```python
from build123d import *

# Parameters (mm, degrees)
SKETCH1_W           = 132
SKETCH1_H           = 160
BOSS_EXTRUDE1_DEPTH = 6
SKETCH3_W           = 32
SKETCH3_H           = 54
SKETCH3_W_2         = 26
SKETCH3_H_2         = 48
BOSS_EXTRUDE2_DEPTH = 17.5
SKETCH4_W           = 32
SKETCH4_H           = 54
BOSS_EXTRUDE3_DEPTH = 3
SKETCH5_W           = 25
SKETCH5_H           = 17
CUT_EXTRUDE1_DEPTH  = 3
SKETCH6_W           = 12
SKETCH6_H           = 54
BOSS_EXTRUDE4_DEPTH = 3
SKETCH7_R           = 1.6
CUT_EXTRUDE2_DEPTH  = 106.177231376
SKETCH8_W           = 3
SKETCH8_H           = 6.5
BOSS_EXTRUDE5_DEPTH = 20
SKETCH9_R           = 1.55
CUT_EXTRUDE3_DEPTH  = 6
SKETCH10_R          = 1.6
CUT_EXTRUDE4_DEPTH  = 108.043215572
SKETCH11_W          = 2.5
SKETCH11_H          = 7
BOSS_EXTRUDE6_DEPTH = 19.36
SKETCH12_R          = 1.6
CUT_EXTRUDE5_DEPTH  = 19.36
SKETCH13_W          = 3
SKETCH13_H          = 7
BOSS_EXTRUDE7_DEPTH = 15
SKETCH14_R          = 2
CUT_EXTRUDE6_DEPTH  = 15
CUT_EXTRUDE7_START  = -6
CUT_EXTRUDE7_DEPTH  = 6
SKETCH16_R          = 1.6
CUT_EXTRUDE8_DEPTH  = 15
CUT_EXTRUDE9_DEPTH  = 69
SKETCH18_W          = 9
SKETCH18_H          = 3
CUT_EXTRUDE10_DEPTH = 69
SKETCH19_R          = 1.55
CUT_EXTRUDE11_DEPTH = 69


# Read off the part's stored shape, not the designer's step: Cut-Extrude7
with BuildPart() as part:
    # Sketch1 → Boss-Extrude1 (new body)
    with BuildSketch(Plane.XY):
        Rectangle(SKETCH1_W, SKETCH1_H)
    extrude(amount=BOSS_EXTRUDE1_DEPTH)

    # Sketch3 → Boss-Extrude2 (add)
    with BuildSketch(Plane.XY.offset(6)):
        with Locations((0, -53)):
            Rectangle(SKETCH3_W, SKETCH3_H)
        with Locations((0, -53)):
            Rectangle(SKETCH3_W_2, SKETCH3_H_2, mode=Mode.SUBTRACT)
    extrude(amount=BOSS_EXTRUDE2_DEPTH)

    # Sketch4 → Boss-Extrude3 (add)
    with BuildSketch(Plane.XY.offset(23.5)):
        with Locations((0, -53)):
            Rectangle(SKETCH4_W, SKETCH4_H)
    extrude(amount=BOSS_EXTRUDE3_DEPTH)

    # Sketch5 → Cut-Extrude1 (cut)
    with BuildSketch(Plane.XZ.offset(80)):
        with Locations((0, 14.5)):
            Rectangle(SKETCH5_W, SKETCH5_H)
    extrude(amount=-CUT_EXTRUDE1_DEPTH, mode=Mode.SUBTRACT)

    # Sketch6 → Boss-Extrude4 (add)
    with BuildSketch(Plane.XY.offset(6)):
        with Locations((-22, -53)):
            Rectangle(SKETCH6_W, SKETCH6_H)
        with Locations((22, -53)):
            Rectangle(SKETCH6_W, SKETCH6_H)
    extrude(amount=BOSS_EXTRUDE4_DEPTH)

    # Sketch7 → Cut-Extrude2 (cut, through all)
    with BuildSketch(Plane.XY.offset(9)):
        with Locations((-22, -69)):
            Circle(SKETCH7_R)
        with Locations((-22, -33)):
            Circle(SKETCH7_R)
        with Locations(Location((22, -69, 0), (0, 0, 180))):
            Circle(SKETCH7_R)
        with Locations(Location((22, -33, 0), (0, 0, 180))):
            Circle(SKETCH7_R)
    extrude(amount=-CUT_EXTRUDE2_DEPTH, mode=Mode.SUBTRACT)

    # Sketch8 → Boss-Extrude5 (add)
    with BuildSketch(Plane.XY.offset(6)):
        with Locations((-54.38, -76.75)):
            Rectangle(SKETCH8_W, SKETCH8_H)
        with Locations((-54.38, -30.25)):
            Rectangle(SKETCH8_W, SKETCH8_H)
    boss_extrude5 = extrude(amount=BOSS_EXTRUDE5_DEPTH)

    # Sketch9 → Cut-Extrude3 (cut)
    with BuildSketch(Plane.ZY.offset(55.88)):
        with Locations((10.35, -76.75)):
            Circle(SKETCH9_R)
        with Locations((19.65, -76.75)):
            Circle(SKETCH9_R)
        with Locations((10.35, -30.25)):
            Circle(SKETCH9_R)
        with Locations((19.65, -30.25)):
            Circle(SKETCH9_R)
    cut_extrude3 = extrude(amount=-CUT_EXTRUDE3_DEPTH, mode=Mode.SUBTRACT)

    # Mirror1: Boss-Extrude5, Cut-Extrude3 across plane
    add(boss_extrude5.mirror(Plane(origin=(0, 0, 0), x_dir=(0, 0, 1), z_dir=(1, 0, 0))))
    add(cut_extrude3.mirror(Plane(origin=(0, 0, 0), x_dir=(0, 0, 1), z_dir=(1, 0, 0))), mode=Mode.SUBTRACT)

    # Sketch10 → Cut-Extrude4 (cut, through all)
    with BuildSketch(Plane(origin=(0, 0, 0), x_dir=(-1, 0, 0), z_dir=(0, 0, -1))):
        with Locations((-24.1, -75.572749788)):
            Circle(SKETCH10_R)
        with Locations((-21.15, -12.732749788)):
            Circle(SKETCH10_R)
        with Locations(Location((21.15, -12.732749788, 0), (0, 0, 180))):
            Circle(SKETCH10_R)
        with Locations((24.1, -75.572749788)):
            Circle(SKETCH10_R)
    extrude(amount=-CUT_EXTRUDE4_DEPTH, mode=Mode.SUBTRACT)

    # Sketch11 → Boss-Extrude6 (add)
    with BuildSketch(Plane(origin=(0, 0, 0), x_dir=(-1, 0, 0), z_dir=(0, 0, -1))):
        with Locations((-17.9, 1.267250212)):
            Rectangle(SKETCH11_W, SKETCH11_H)
        with Locations((-17.9, 50.267250212)):
            Rectangle(SKETCH11_W, SKETCH11_H)
    extrude(amount=BOSS_EXTRUDE6_DEPTH)

    # Sketch12 → Cut-Extrude5 (cut)
    with BuildSketch(Plane(origin=(19.15, 0, 0), x_dir=(0, 0, -1), z_dir=(1, 0, 0))):
        with Locations(Location((4.5, 50.267250212, 0), (0, 0, 90))):
            Circle(SKETCH12_R)
        with Locations(Location((14.5, 50.267250212, 0), (0, 0, 90))):
            Circle(SKETCH12_R)
        with Locations(Location((4.5, 1.267250212, 0), (0, 0, 90))):
            Circle(SKETCH12_R)
        with Locations(Location((14.5, 1.267250212, 0), (0, 0, 90))):
            Circle(SKETCH12_R)
    extrude(amount=-CUT_EXTRUDE5_DEPTH, mode=Mode.SUBTRACT)

    # Sketch13 → Boss-Extrude7 (add)
    with BuildSketch(Plane(origin=(0, 0, 0), x_dir=(-1, 0, 0), z_dir=(0, 0, -1))):
        with Locations((29.35, 35.967250212)):
            Rectangle(SKETCH13_W, SKETCH13_H)
    extrude(amount=BOSS_EXTRUDE7_DEPTH)

    # Sketch14 → Cut-Extrude6 (cut)
    with BuildSketch(Plane.ZY.offset(30.85)):
        with Locations((-9.9, 35.967250212)):
            Circle(SKETCH14_R)
    extrude(amount=-CUT_EXTRUDE6_DEPTH, mode=Mode.SUBTRACT)

    # Cut-Extrude7 outline → Cut-Extrude7 (cut)
    with BuildSketch(Plane(origin=(0, 0, 0), x_dir=(-1, 0, 0), z_dir=(0, 0, -1)).offset(CUT_EXTRUDE7_START)):
        Polygon((-30.85, 56.767250212), (30.85, 56.767250212), (30.85, -24), (58.88, -24), (58.88, -80), (66, -80), (66, 80), (-66, 80), (-66, -80), (-58.88, -80), (-58.88, -24), (-30.85, -24), align=None)
    extrude(amount=CUT_EXTRUDE7_DEPTH, mode=Mode.SUBTRACT)

    # Sketch16 → Cut-Extrude8 (cut)
    with BuildSketch(Plane(origin=(0, 0, 0), x_dir=(-1, 0, 0), z_dir=(0, 0, -1))):
        Circle(SKETCH16_R)
        with Locations((0, 52.767250212)):
            Circle(SKETCH16_R)
    extrude(amount=-CUT_EXTRUDE8_DEPTH, mode=Mode.SUBTRACT)

    # Sketch17 → Cut-Extrude9 (cut)
    with BuildSketch(Plane(origin=(0, 0, 0), x_dir=(-1, 0, 0), z_dir=(0, 0, -1))):
        Polygon((-30.85, 56.767250212), (30.85, 56.767250212), (30.85, 39.467250212), (18.85, 39.467250212), (18.85, 32.467250212), (30.85, 32.467250212), (58.88, -24), (58.88, -80), (-58.88, -80), (-58.88, 56.767250212), align=None)
    extrude(amount=-CUT_EXTRUDE9_DEPTH, mode=Mode.SUBTRACT)


with BuildPart() as body_2:
    # of the pieces the cut leaves, the one that is kept (cut_extrude9_keep)
    add(part.part.solids().sort_by_distance((-27.85, 39.467250212, 0))[0])

    # Sketch18 → Cut-Extrude10 (cut)
    with BuildSketch(Plane.XZ.offset(-32.467250212)):
        with Locations((-23.35, 1.5)):
            Rectangle(SKETCH18_W, SKETCH18_H)
    extrude(amount=-CUT_EXTRUDE10_DEPTH, mode=Mode.SUBTRACT)

    # Sketch19 → Cut-Extrude11 (cut)
    with BuildSketch(Plane(origin=(0, 0, 3), x_dir=(-1, 0, 0), z_dir=(0, 0, -1))):
        with Locations((22.35, 35.967250212)):
            Circle(SKETCH19_R)
    extrude(amount=-CUT_EXTRUDE11_DEPTH, mode=Mode.SUBTRACT)


solid = body_2.part
```
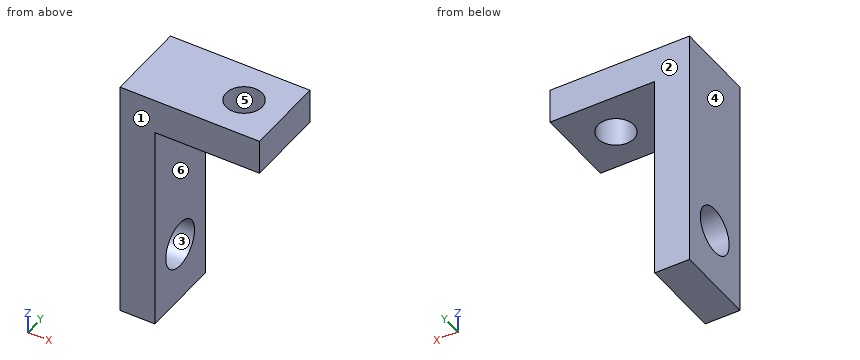
Input: part model. Units: mm. Frame: model coordinates. Face numbers are marked on the shaded views. A direction names the side the tool comes from. Coordinates: 2 decimals unless noted, no trailing zeros. Write each loop counter-clockwise with the first axis right and the second up, starting at its lowest first coordinate (ties: lowest second). Pieces come first, ordered by that corner, then holes. Notation, with made-up numbers: (80.5, 85.25) -> (122.5, 85.25) arc R14 ccw to (122.5, 104.25) -> close; hole circle Ø5 at (12.5, 78). An arc over 180 degrees is marked (long way). Write each question's results on one line, items separated by ' | '.
Item 1: Section query A-A on x = -22.35. Return loops of the section in (y, z), plus the area to 3 significant figures.
Conclusion:
outline: (32.47, 3) -> (34.42, 3) -> (34.42, 6) -> (32.47, 6) -> close; (37.52, 3) -> (39.47, 3) -> (39.47, 6) -> (37.52, 6) -> close | area: 11.7 mm^2
Item 2: Mould query, pull axis Y, two halves, no side actions, for the marked faces 1, 2, 3 and 4. Classes: +Y half, -Y half, draft (parallel to the pull), parting line (faces both ways), or undercut.
Conclusion:
face 1: -Y half | face 2: +Y half | face 3: undercut | face 4: draft
Item 3: Section query D-D on z = 4.75. Return loops of the section in (x, y).
Conclusion:
outline: (-30.85, 32.47) -> (-18.85, 32.47) -> (-18.85, 39.47) -> (-30.85, 39.47) -> close; hole circle Ø3.1 at (-22.35, 35.97)
Item 4: Pin query (flat end, axial travel): pin 1 Ø3.5 at (x, y) = (-22.35, 35.97) entering from -Z. Return the tip coordinate at first contact, or that it passes through.
Conclusion:
pin 1: stops at z = 3
Item 5: Section query C-C on y = 33. Return loops of the section in (x, z).
Conclusion:
outline: (-30.85, -15) -> (-27.85, -15) -> (-27.85, 3) -> (-18.85, 3) -> (-18.85, 6) -> (-30.85, 6) -> close
Item 6: Material intervals for probe 1 along Y at (x, z) = (-22.35, 4.65); probe 2 along Y at (x, z) = (-28.5, -9.9); probe 3 along Z at (x, y) = (-20, 37.25), sorted ascending.
Conclusion:
probe 1: y = 32.47 to 34.42, 37.52 to 39.47 | probe 2: y = 32.47 to 33.97, 37.97 to 39.47 | probe 3: z = 3 to 6
Item 7: Set-up query: the marked faces 5 and 6. Return all of +Z, -Z, +X, -X, +Y, -Y with unobstructed straight access to the full face (end or side cutting, diameter ignored); none if empty.
Conclusion:
face 5: +Z, -Z | face 6: -Z, +X, +Y, -Y
Item 8: Section query B-B on z = -9.9. Return loops of the section in (x, y), plus the area to 3 significant figures.
Conclusion:
outline: (-30.85, 32.47) -> (-27.85, 32.47) -> (-27.85, 33.97) -> (-30.85, 33.97) -> close; (-30.85, 37.97) -> (-27.85, 37.97) -> (-27.85, 39.47) -> (-30.85, 39.47) -> close | area: 9.00 mm^2
